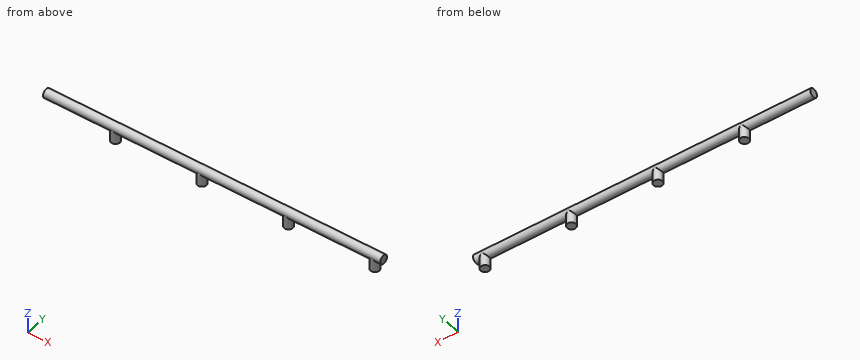
```python
from build123d import *

# Parameters (mm, degrees)
F0_R      = 12.7
F1_DEPTH  = 1200
F2_R      = 12.7
F3_DEPTH  = 40
F1_FACE_R = 12.7
F4_DEPTH  = 225


with BuildPart() as f1:
    # F0 (on Right) → F1 (new body)
    with BuildSketch(Plane.YZ):
        Circle(F0_R)
    extrude(amount=-F1_DEPTH)

    # F2 (on Top) → F3 (join)
    with BuildSketch(Plane.XY):
        with Locations((-250, 0)):
            Circle(F2_R)
        with Locations((-500, 0)):
            Circle(F2_R)
        with Locations((-750, 0)):
            Circle(F2_R)
        with Locations((-1000, 0)):
            Circle(F2_R)
    extrude(amount=-F3_DEPTH)

    # F1_face (on face) → F4 (cut)
    with BuildSketch(Plane.YZ):
        Circle(F1_FACE_R)
    extrude(amount=-F4_DEPTH, mode=Mode.SUBTRACT)


solid = f1.part
```
The model under review builds one solid part; all positions refer to its coordinate system, in mm. Round coordinates to 2 decimals unless told otherwise and drop trailing zeros. Loops run counter-clockwise (first coordinate to the right, second up) from the corner with the lowest first, then second, coordinate; pieces in that order, holes last.
Item 1: Clearance check with flat-ended pins moving along their axes: pin 1 Ø5 at (y, z) = (-9, -15.5) entering from -X; pin 2 Ø5 at (y, z) = (8.5, -10.5) entering from -X; pin 3 Ø5 at (y, z) = (-1, -15.5) entering from +X; pin 4 Ø3 at (x, y) = (-918, 1) entering from -Z. State where each tip first meets the part, or that it passes through.
Determined:
pin 1: stops at x = -1010.91
pin 2: stops at x = -1200
pin 3: stops at x = -237.3
pin 4: stops at z = -12.7
Item 2: Take a section at A-A (y = 0). Write out the cut boundary in (x, z).
Determined:
outline: (-1200, -12.7) - (-1012.7, -12.7) - (-1012.7, -40) - (-987.3, -40) - (-987.3, -12.7) - (-762.7, -12.7) - (-762.7, -40) - (-737.3, -40) - (-737.3, -12.7) - (-512.7, -12.7) - (-512.7, -40) - (-487.3, -40) - (-487.3, -12.7) - (-262.7, -12.7) - (-262.7, -40) - (-237.3, -40) - (-237.3, -12.7) - (-225, -12.7) - (-225, 12.7) - (-1200, 12.7) - close
Item 3: For line 1 (X direction, y = -4.5, z = -34); line 2 (X direction, y = -2.25, z = -38); line 3 (Z direction, x = -531.5, y = 0), list the stretches that pass through material, from the lowest coordinate up.
Determined:
line 1: x = -1011.88 to -988.12, -761.88 to -738.12, -511.88 to -488.12, -261.88 to -238.12
line 2: x = -1012.5 to -987.5, -762.5 to -737.5, -512.5 to -487.5, -262.5 to -237.5
line 3: z = -12.7 to 12.7
Item 4: Take a section at D-D (x = -656). Write out the cut boundary in (y, z).
Determined:
outline: circle Ø25.4 at (0, 0)
Item 5: Take a section at B-B (z = -28). Write out the cut boundary in (x, y), then the cut area to 3 significant figures.
Determined:
outline: circle Ø25.4 at (-1000, 0); circle Ø25.4 at (-750, 0); circle Ø25.4 at (-500, 0); circle Ø25.4 at (-250, 0)
area: 2,030 mm2
Item 6: Take a section at C-C (x = -500). Write out the cut boundary in (y, z).
Determined:
outline: (-12.7, -40) - (12.7, -40) - (12.7, 0) arc R12.7 ccw to (-12.7, 0) - close
